CAD build for the part. Positions are in the model's coordinates, mm. Face numbers are marked on the shaded views. Coordinates: 2 decimals unless noted, no trailing zeros. Order: outer loops, then holes, each group sorted by start corner. A loop starts at its lowest first (then second) coordinate and runs counter-clockwise, first axis right, second up. Notation, with made-up numbers: (36.25, 89) - (84.25, 89) arc R18 ccw to (84.25, 113) - close; hole circle Ø6 at (33, -10). An arc over 180 degrees is marked (long way). Return JSON: item names as keys, results as strings.
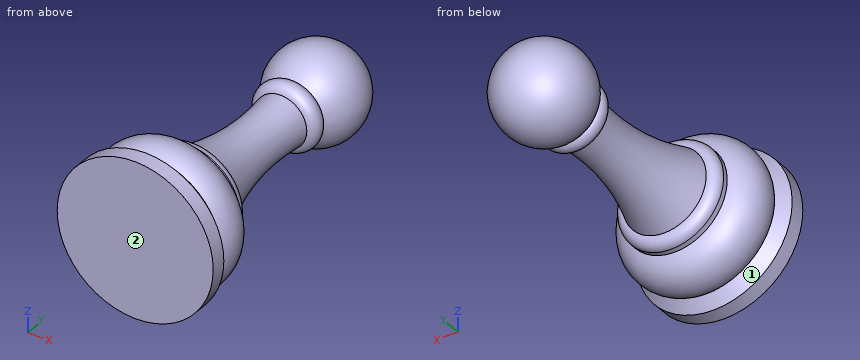
from build123d import *


with BuildPart() as part:
    # Sketch1 → Revolve3 (revolve)
    with BuildSketch(Plane.XY, mode=Mode.PRIVATE) as revolve3_sk:
        with BuildLine():
            Line((0, 0), (-15, 0))
            Line((-15, 0), (-15, 3))
            Line((-15, 3), (-13, 5))
            ThreePointArc((-13, 5), (-13.688325627, 10.216881481), (-10, 13.97))
            Line((-10, 13.97), (-10, 14.97))
            ThreePointArc((-10, 14.97), (-9.414213562, 16.384213562), (-8, 16.97))
            ThreePointArc((-8, 16.97), (-5.019495729, 28.81539847), (-5, 41.03))
            ThreePointArc((-5, 41.03), (-6.412519214, 42.380086131), (-6, 44.29))
            ThreePointArc((-6, 44.29), (-8.408390155, 54.210585037), (0, 60))
            Line((0, 60), (0, 0))
        make_face()
    revolve(revolve3_sk.sketch.rotate(Axis((0, 0, 0), (0, 1, 0)), 180), axis=Axis((0, 0, 0), (0, 1, 0)))


solid = part.part
Item 1: Mould opens along Y. For the marked faces 1 and 2 say: released by +Y, released by -Y, zero draft, split by the parting line, or undercut.
Findings below:
{"face 1": "undercut", "face 2": "released by -Y"}
Item 2: Band-saw the part on B-B, the plane z = 0. List the corners of the cut face in (x, y), then the cut area to 3 significant figures.
Findings below:
{"outline": "(-15, 0) - (15, 0) - (15, 3) - (13, 5) arc R6 ccw to (10, 13.97) - (10, 14.97) arc R2 ccw to (8, 16.97) arc R50 cw to (5, 41.03) arc R2 ccw to (6, 44.29) arc R9 ccw (long way) to (-6, 44.29) arc R2 ccw to (-5, 41.03) arc R50 cw to (-8, 16.97) arc R2 ccw to (-10, 14.97) - (-10, 13.97) arc R6 ccw to (-13, 5) - (-15, 3) - close", "area": "982 mm²"}
Item 3: Wall check: L1, parallel to Y at x = -11.5, z = 7.25; L2, parallel to Z at x = -8, y = 49; L3, parallel to X at y = 34.5, z = 3.75. Give the ranges that are in metal, low to high. Write a range as [from, to].
Findings below:
{"L1": "y = [0, 4.41], [6.15, 10.48]", "L2": "z = [-3.61, 3.61]", "L3": "x = [-2.73, 2.73]"}
Item 4: Band-saw the part on C-C, the plane y = 48. List the corners of the cut face in (x, z), then the cut area to 3 significant figures.
Findings below:
{"outline": "circle Ø16.97 at (0, 0)", "area": "226 mm²"}
Item 5: Band-saw the part on A-A, the plane x = 0. List the corners of the cut face in (y, z), then the cut area to 3 significant figures.
Findings below:
{"outline": "(0, -15) - (3, -15) - (5, -13) arc R6 ccw to (13.97, -10) - (14.97, -10) arc R2 ccw to (16.97, -8) arc R50 cw to (41.03, -5) arc R2 ccw to (44.29, -6) arc R9 ccw (long way) to (44.29, 6) arc R2 ccw to (41.03, 5) arc R50 cw to (16.97, 8) arc R2 ccw to (14.97, 10) - (13.97, 10) arc R6 ccw to (5, 13) - (3, 15) - (0, 15) - close", "area": "982 mm²"}
Item 6: Drop flat-ended pins along their axis: P1, Ø6, axis at x = -6, y = 23.5, coming from the +Z side; P2, Ø3, axis at x = -5, y = 39, coming from the -Z side; P3, Ø6, axis at x = 1, z = 10, coming from the +Y side. Give the stop position or say it passes through.
Findings below:
{"P1": "stops at z = 5.37", "P2": "stops at z = -3.29", "P3": "stops at y = 56.6"}
